from build123d import *

# Parameters (mm, degrees)
SKETCH3_R          = 1.5
CUT_EXTRUDE1_DEPTH = 4


with BuildPart() as part:
    # Sketch2 → Revolve1 (revolve)
    with BuildSketch(Plane(origin=(0, 0, 0), x_dir=(1, 0, 0), z_dir=(0, 1, 0))):
        Polygon((0, 0), (0, 15), (-2.7, 15), (-2.7, 20), (-19.2, 20), (-19.2, 21), (-20.7, 21), (-20.7, 17.652837292), (-20.7, 14.5), (-20.7, 8), (-15.7, 8), (-15.7, 6), (-14.7, 6), (-14.7, 0), align=None)
    revolve(axis=Axis((0, 0, 0), (-1, 0, 0)))

    # Sketch3 → Cut-Extrude1 (cut)
    with BuildSketch(Plane.ZY.offset(20.7)):
        with Locations((0, 16)):
            Circle(SKETCH3_R)
        with Locations((13.856406461, 7.904729806)):
            Circle(SKETCH3_R)
        with Locations((13.773900052, -8.142905292)):
            Circle(SKETCH3_R)
        with Locations((-0.165012817, -16.095270194)):
            Circle(SKETCH3_R)
        with Locations((-14.021419278, -8)):
            Circle(SKETCH3_R)
        with Locations((-13.938912869, 8.047635097)):
            Circle(SKETCH3_R)
    extrude(amount=-CUT_EXTRUDE1_DEPTH, mode=Mode.SUBTRACT)


solid = part.part
The listing builds one solid part. Answer for the finished solid, in the listing's coordinates (mm). A direction names the side the tool comes from. Coordinates: 2 decimals unless noted, no trailing zeros. Loops run counter-clockwise (first coordinate to the right, second up) from the corner with the lowest first, then second, coordinate; pieces in that order, holes last. Notation, with made-up numbers: (81, -22) -> (103, -22) arc R21 cw to (103, -10) -> close; hole circle Ø5 at (60.5, -19.75). An arc over 180 degrees is marked (long way). Write item = value, one per line. Start each with the question number.
1) The mould has two halves that part along Y. Classify faces 1 (the face through (-20.7, 0, -9)), 2 (the face through (-18.728, -6.656, 13.579)), 3 (the face through (-19.96, -6.31, -20.03)): released by +Y, released by -Y, zero draft, split by the parting line, or undercut.
2) A cutting plane is placed at B-B (z = -3.5). Give the vertices of the cut face in (x, y).
3) A tool of negligible diameter and unlimited length cuts with its end or side. For faces 4 (the face through (-16.7, 8, 14)), 5 (the face through (-19.2, 8, 19)), 6 (the face through (0, 0, 0)), from which of +Z, -Z, +X, -X, +Y, -Y can it reach the whole face along a straight path? Write none if from no direction.
4) Straight lines are drawn through the part: line 1 (Y direction, x = -18.3, z = 0); line 2 (Z direction, x = -18.7, y = 0); line 3 (X direction, y = -19, z = -8). For each, find the intervals that lie inside material, in ascending order. Write a range as from..to.
5) A cutting plane is placed at C-C (y = -13). Give the vertices of the cut face in (x, z), then the cut area to 3 significant figures.
6) A cutting plane is placed at A-A (y = 0). Give the vertices of the cut face in (x, z).
7) Given pin 1 Ø1.5 at (y, z) = (-16.5, -0.5) entering from -X; pin 2 Ø2 at (x, z) = (-4.5, -7) entering from +Y; pin 3 Ø1 at (x, y) = (-17, -8.5) entering from +Z, each flat-ended and moving along its own axis, determine where each tip first touches the part or whether it passes through.
8) A cutting plane is placed at D-D (z = 11). Give the vertices of the cut face in (x, y).
Responses:
q1.face_1 = zero draft
q1.face_2 = undercut
q1.face_3 = split by the parting line
q2.outline = (-20.7, -20.71) -> (-19.2, -20.71) -> (-19.2, -19.69) -> (-2.7, -19.69) -> (-2.7, -14.59) -> (0, -14.59) -> (0, 14.59) -> (-2.7, 14.59) -> (-2.7, 19.69) -> (-19.2, 19.69) -> (-19.2, 20.71) -> (-20.7, 20.71) -> (-20.7, 7.19) -> (-15.7, 7.19) -> (-15.7, 4.87) -> (-14.7, 4.87) -> (-14.7, -4.87) -> (-15.7, -4.87) -> (-15.7, -7.19) -> (-20.7, -7.19) -> close
q3.face_4 = -X
q3.face_5 = +X
q3.face_6 = +Z, -Z, +X, +Y, -Y
q4.line_1 = -20..-17.59, -14.6..-8, 8..14.5, 17.5..20
q4.line_2 = -20..-8, 8..20
q4.line_3 = -20.7..-19.2
q5.outline = (-20.7, -16.49) -> (-19.2, -16.49) -> (-19.2, -15.2) -> (-2.7, -15.2) -> (-2.7, -7.48) -> (0, -7.48) -> (0, 7.48) -> (-2.7, 7.48) -> (-2.7, 15.2) -> (-19.2, 15.2) -> (-19.2, 16.49) -> (-20.7, 16.49) -> close
q5.area = 591 mm²
q6.outline = (-20.7, -21) -> (-19.2, -21) -> (-19.2, -20) -> (-2.7, -20) -> (-2.7, -15) -> (0, -15) -> (0, 15) -> (-2.7, 15) -> (-2.7, 20) -> (-19.2, 20) -> (-19.2, 21) -> (-20.7, 21) -> (-20.7, 8) -> (-15.7, 8) -> (-15.7, 6) -> (-14.7, 6) -> (-14.7, -6) -> (-15.7, -6) -> (-15.7, -8) -> (-20.7, -8) -> close
q7.pin_1 = -16.7
q7.pin_2 = 19.08
q7.pin_3 = 18.33
q8.outline = (-20.7, -17.89) -> (-19.2, -17.89) -> (-19.2, -16.7) -> (-2.7, -16.7) -> (-2.7, -10.2) -> (0, -10.2) -> (0, 10.2) -> (-2.7, 10.2) -> (-2.7, 16.7) -> (-19.2, 16.7) -> (-19.2, 17.89) -> (-20.7, 17.89) -> close
